Source: CAD feature listing. Evaluate the final solid. Frame: model axes, mm. A direction names the side the tool comes from. Round coordinates to 2 decimals unless told otherwise and drop trailing zeros. Write each loop counter-clockwise with the first axis right and the second up, starting at its lowest first coordinate (ties: lowest second). Pieces come first, ordered by that corner, then holes. Notation, with made-up numbers: M 50.5,-26.75 L 62.5,-26.75 A22 ccw 62.5,-9.75 Z; hole C 52.5,14.5 d5. An arc over 180 degrees is marked long. Use a Markdown table: item, result.
```python
from build123d import *

# Parameters (mm, degrees)
SKETCH_1_R          = 3
EXTRUDE_1_DEPTH     = 13
SKETCH_2_R          = 1.5
EXTRUDE_2_DEPTH     = 5
CHAMFER_1_SIZE      = 0.5
SKETCH_3_R          = 1.5
SKETCH_3_R_2        = 1.25
CUT_EXTRUDE_3_DEPTH = 1.5
SKETCH_4_W          = 2
SKETCH_4_H          = 2
CUT_EXTRUDE_4_DEPTH = 10
CHAMFER_2_SIZE      = 0.5


with BuildPart() as part:
    # 草图1 → 拉伸1 (new body)
    with BuildSketch(Plane.XY):
        with Locations(Location((0, 0, 0), (0, 0, 180))):
            Circle(SKETCH_1_R)
    extrude(amount=EXTRUDE_1_DEPTH)

    # 草图2 → 拉伸2 (add)
    with BuildSketch(Plane.XY.offset(13)):
        Circle(SKETCH_2_R)
    extrude(amount=EXTRUDE_2_DEPTH)

    # 倒角1
    chamfer_1_edges = [part.edges().sort_by_distance(p)[0] for p in [
        (-1.5, 0, 18),
    ]]
    chamfer(chamfer_1_edges, length=CHAMFER_1_SIZE)

    # 草图3 → 拉伸3 (cut)
    with BuildSketch(Plane.XY.offset(13)):
        Circle(SKETCH_3_R)
        Circle(SKETCH_3_R_2, mode=Mode.SUBTRACT)
    extrude(amount=CUT_EXTRUDE_3_DEPTH, mode=Mode.SUBTRACT)

    # 草图4 → 拉伸4 (cut, symmetric)
    with BuildSketch(Plane(origin=(0, 0, 0), x_dir=(0, 0, -1), z_dir=(1, 0, 0))):
        with Locations((-1, 0)):
            Rectangle(SKETCH_4_W, SKETCH_4_H)
    extrude(amount=CUT_EXTRUDE_4_DEPTH, both=True, mode=Mode.SUBTRACT)

    # 倒角2
    chamfer_2_edges = [part.edges().sort_by_distance(p)[0] for p in [
        (0, 3, 0),
        (0, -3, 0),
        (3, 0, 13),
    ]]
    chamfer(chamfer_2_edges, length=CHAMFER_2_SIZE)


solid = part.part
```
Q1. Section D-D on z = 13.5. Return loops of the section in (x, y).
Results are:
| item | result |
|---|---|
| outline | C 0,0 d2.5 |
Q2. Mould query, pull axis Y, two halves, no side actions, for faces 6 (the cylindrical face through (-1.384, 2.662, 6.416)), 7 (the flat face through (0, 0, 2)), 8 (the flat face through (0, 2, 0)). Classes: +Y half, -Y half, draft (parallel to the pull), parting line (faces both ways), or undercut.
Results are:
| item | result |
|---|---|
| face 6 | parting line |
| face 7 | undercut |
| face 8 | draft |
Q3. Reachability of faces 1 (the conical face through (0.045, 2.635, 0.135)), 2 (the flat face through (0, -1, 1)), 3 (the cylindrical face through (-1.5, 0.07, 15.98)), 4 (the cylindrical face through (-0.27, -1.22, 13.74)), 5 (the conical face through (-0.045, -2.635, 0.135)) from +Z, -Z, +X, -X, +Y, -Y: full face, straight path, thin tool, end or side. Return the list, or none.
Results are:
| item | result |
|---|---|
| face 1 | -Z, +Y |
| face 2 | -Z, +X, -X |
| face 3 | +Z |
| face 4 | none |
| face 5 | -Z, -Y |
Q4. Section C-C on z = 8. Return loops of the section in (x, y).
Results are:
| item | result |
|---|---|
| outline | C 0,0 d6 |
Q5. Line query: L1, parallel to Z at x = 1.6, y = 1.8; L2, parallel to Z at x = -1.95, y = 0.3; L3, parallel to Y at x = 1.65, z = 1. Output: solid intervals per line, ascending.
Results are:
| item | result |
|---|---|
| L1 | 0 to 13 |
| L2 | 2 to 13 |
| L3 | -2.51 to -1, 1 to 2.51 |
Q6. First-contact query: pin 1 Ø2 at (y, z) = (1.5, 9) entering from +X; pin 2 Ø1 at (x, y) = (1, 0) entering from -Z; pin 3 Ø1 at (x, z) = (-1, 16) entering from -Y. Flat tips, straight axial feed; report the tip coordinate or a pass-through.
Results are:
| item | result |
|---|---|
| pin 1 | x = 2.96 |
| pin 2 | z = 2 |
| pin 3 | y = -1.41 |
Q7. Section B-B on y = 0. Return loops of the section in (x, z).
Results are:
| item | result |
|---|---|
| outline | M -3,2 L 3,2 L 3,12.5 L 2.5,13 L 1.25,13 L 1.25,14.5 L 1.5,14.5 L 1.5,17.5 L 1,18 L -1,18 L -1.5,17.5 L -1.5,14.5 L -1.25,14.5 L -1.25,13 L -2.5,13 L -3,12.5 Z |
Q8. Section A-A on x = 0. Return loops of the section in (y, z).
Results are:
| item | result |
|---|---|
| outline | M -3,0.5 L -2.5,0 L -1,0 L -1,2 L 1,2 L 1,0 L 2.5,0 L 3,0.5 L 3,12.5 L 2.5,13 L 1.25,13 L 1.25,14.5 L 1.5,14.5 L 1.5,17.5 L 1,18 L -1,18 L -1.5,17.5 L -1.5,14.5 L -1.25,14.5 L -1.25,13 L -2.5,13 L -3,12.5 Z |
